from build123d import *

# Parameters (mm, degrees)
ESQUISSE1_W             = 40
ESQUISSE1_H             = 35
ESQUISSE1_W_2           = 12
ESQUISSE1_H_2           = 2.5
BOSS_EXTRU_1_DEPTH      = 2
ENL_V_MAT_EXTRU_1_DEPTH = 10


with BuildPart() as part:
    # Esquisse1 → Boss.-Extru.1 (new body)
    with BuildSketch(Plane(origin=(0, 0, 0), x_dir=(1, 0, 0), z_dir=(0, 1, 0))):
        Rectangle(ESQUISSE1_W, ESQUISSE1_H)
        with BuildLine():
            Line((6.15, 1.220085228), (6.15, 0))
            ThreePointArc((6.15, 0), (9, -2.85), (11.85, 0))
            Line((11.85, 0), (11.85, 1.220085228))
            ThreePointArc((11.85, 1.220085228), (9, 12.5), (6.15, 1.220085228))
        make_face(mode=Mode.SUBTRACT)
        with Locations((-9, 11.25)):
            Rectangle(ESQUISSE1_W_2, ESQUISSE1_H_2, mode=Mode.SUBTRACT)
    extrude(amount=BOSS_EXTRU_1_DEPTH)

    # Esquisse2 → Enlèv. mat.-Extru.1 (cut)
    with BuildSketch(Plane(origin=(0, 2, 0), x_dir=(1, 0, 0), z_dir=(0, 1, 0))):
        with BuildLine():
            Line((-24.036917244, 12.452787924), (-23.501994654, -22.917521082))
            Line((-23.501994654, -22.917521082), (20, -17.5))
            add(Edge.make_bspline(
                [(20, -17.5), (-13.836799154, -13.898150417), (-24.036917244, 12.452787924)],
                knots=[0, 0, 0, 1, 1, 1], degree=2))
        make_face()
    extrude(amount=-ENL_V_MAT_EXTRU_1_DEPTH, mode=Mode.SUBTRACT)


solid = part.part
Work out the finished part from the listing and answer in its coordinate system (mm). A direction names the side the tool comes from. Give positions to 0.01 mm unless a question says otherwise; leave off trailing zeros. Write each loop counter-clockwise with the first axis right and the second up, starting at its lowest first coordinate (ties: lowest second). Pieces come first, ordered by that corner, then holes.
Q1. A tool of negligible diameter and unlimited length cuts with its end or side. For faces 4 (the face through (4, 0, 0)), 5 (the face through (-3, 1, -11)), from which of +Z, -Z, +X, -X, +Y, -Y can it reach the whole face along a straight path? Write none if from no direction.
Answer:
face 4: +Z, -Z, +X, -X, -Y
face 5: +Y, -Y
Q2. Straight lines are drawn through the part: L1, parallel to X at y = 1.35, z = -6.5; L2, parallel to Z at x = -6, y = 1.95; L3, parallel to X at y = 1.05, z = -9. For each, find the intervals that lie inside material, in ascending order.
Answer:
L1: x = -20 to 3, 15 to 20
L2: z = -17.5 to -12.5, -10 to 9.45
L3: x = -20 to 3.55, 14.45 to 20
Q3. Given pin 1 (12 mm diameter, centred on x = 5.5, z = -9.5, fed in from -Y); pin 2 (7 mm diameter, centred on x = 9, z = -6.5, fed in from +Y); pin 3 (0.6 mm diameter, centred on y = 1, z = -0.5, fed in from -X), each flat-ended and moving along its own axis, determine where each tip first touches the part or whether it passes through.
Answer:
pin 1: stops at y = 0
pin 2: passes through
pin 3: stops at x = -17.54
Q4. The part is cut by section A-A on z = -6.5. Give the vertices of the cut face in (x, y), and give its area (3 significant figures).
Answer:
outline: (-20, 0) - (3, 0) - (3, 2) - (-20, 2) - close; (15, 0) - (20, 0) - (20, 2) - (15, 2) - close
area: 56.0 mm2
Q5. For a pull along X with two mould halves and no side action, classify faces 1 (the face through (-20, 1, -11)), 2 (the face through (0, 1, -17.5)), 3 (the face through (-15, 1, -11)) as released by +X, released by -X, zero draft, split by the parting line, or undercut.
Answer:
face 1: released by -X
face 2: zero draft
face 3: undercut
Q6. The part is cut by section B-B on y = 0.5. State how many separate pieces and enclosed holes the cut face has, and give its area (3 significant figures).
Answer:
separate pieces: 1
enclosed holes: 2
area: 969 mm2
